```python
from build123d import *

# Parameters (mm, degrees)
SKETCH_3_W           = 2
SKETCH_3_H           = 46.5
SKETCH_5_W           = 2
SKETCH_5_H           = 46.5
SKETCH_6_R           = 9.5
CUT_EXTRUDE_1_DEPTH  = 328.171973127
SKETCH_7_R           = 9.5
CUT_EXTRUDE_2_DEPTH  = 328.171973127
SKETCH_8_R           = 9.5
CUT_EXTRUDE_3_DEPTH  = 328.171973127
SKETCH_9_R           = 9.5
CUT_EXTRUDE_4_DEPTH  = 328.171973127
SKETCH_10_R          = 9.5
CUT_EXTRUDE_5_DEPTH  = 328.171973127
SKETCH_11_R          = 9.5
CUT_EXTRUDE_6_DEPTH  = 328.171973127
SKETCH_12_R          = 9.5
CUT_EXTRUDE_7_DEPTH  = 328.171973127
SKETCH_13_R          = 9.5
CUT_EXTRUDE_8_DEPTH  = 328.171973127
SKETCH_14_R          = 9.5
CUT_EXTRUDE_9_DEPTH  = 328.171973127
SKETCH_15_R          = 9.5
CUT_EXTRUDE_10_DEPTH = 328.171973127
SKETCH_16_R          = 9.5
CUT_EXTRUDE_11_DEPTH = 328.171973127
SKETCH_17_R          = 9.5
CUT_EXTRUDE_12_DEPTH = 328.171973127
SKETCH_18_R          = 6
CUT_EXTRUDE_13_DEPTH = 328.171973127


with BuildPart() as part:
    # Эскиз1 → Повернуть1 (revolve)
    with BuildSketch(Plane.XY, mode=Mode.PRIVATE) as revolve_1_sk:
        with BuildLine():
            Line((0, 0), (273, 0))
            Line((273, 0), (273, 98.4))
            Line((273, 98.4), (271.4, 100))
            Line((271.4, 100), (265, 100))
            Line((265, 100), (265, 127.5))
            Line((265, 127.5), (247, 127.5))
            Line((247, 127.5), (247, 100))
            Line((247, 100), (239, 100))
            Line((239, 100), (239, 62.5))
            Line((239, 62.5), (218, 62.5))
            Line((218, 62.5), (215, 60.767949192))
            Line((215, 60.767949192), (215, 57))
            ThreePointArc((215, 57), (214.414213562, 55.585786438), (213, 55))
            Line((213, 55), (183, 55))
            Line((183, 55), (178.669872981, 52.5))
            Line((178.669872981, 52.5), (95, 52.5))
            Line((95, 52.5), (95, 50))
            Line((95, 50), (42, 50))
            Line((42, 50), (42, 45))
            Line((42, 45), (0, 45))
            Line((0, 45), (0, 0))
        make_face()
    revolve(revolve_1_sk.sketch.rotate(Axis((0, 0, 0), (1, 0, 0)), 90), axis=Axis((0, 0, 0), (1, 0, 0)))

    # Эскиз2 → Вырез-Повернуть1 (revolve, cut)
    with BuildSketch(Plane.XY, mode=Mode.PRIVATE) as cut_revolve_1_sk:
        Polygon((0, 0), (273, 0), (273, 95), (265, 95), (265, 45), (254, 45), (254, 39), (240, 39), (240, 34), (203.5, 34), (203.5, 31), (0, 31), align=None)
    revolve(cut_revolve_1_sk.sketch.rotate(Axis((0, 0, 0), (1, 0, 0)), 90), axis=Axis((0, 0, 0), (1, 0, 0)), mode=Mode.SUBTRACT)

    # Эскиз3 → Rear_recess_left (revolve, cut)
    with BuildSketch(Plane.XY, mode=Mode.PRIVATE) as rear_recess_left_sk:
        with Locations((261, 71.75)):
            Rectangle(SKETCH_3_W, SKETCH_3_H)
    revolve(rear_recess_left_sk.sketch.rotate(Axis((0, 0, 0), (1, 0, 0)), 90), axis=Axis((0, 0, 0), (1, 0, 0)), mode=Mode.SUBTRACT)

    # Эскиз4 → Collar_groove_nominal (revolve, cut)
    with BuildSketch(Plane.XY, mode=Mode.PRIVATE) as collar_groove_nominal_sk:
        with BuildLine():
            Line((263, 48), (263, 95))
            Line((263, 95), (262, 95))
            Line((262, 95), (262, 48))
            ThreePointArc((262, 48), (262.146446609, 47.646446609), (262.5, 47.5))
            ThreePointArc((262.5, 47.5), (262.853553391, 47.646446609), (263, 48))
        make_face()
    revolve(collar_groove_nominal_sk.sketch.rotate(Axis((0, 0, 0), (1, 0, 0)), 90), axis=Axis((0, 0, 0), (1, 0, 0)), mode=Mode.SUBTRACT)

    # Эскиз5 → Rear_recess_lip (revolve, cut)
    with BuildSketch(Plane.XY, mode=Mode.PRIVATE) as rear_recess_lip_sk:
        with Locations((264, 71.75)):
            Rectangle(SKETCH_5_W, SKETCH_5_H)
    revolve(rear_recess_lip_sk.sketch.rotate(Axis((0, 0, 0), (1, 0, 0)), 90), axis=Axis((0, 0, 0), (1, 0, 0)), mode=Mode.SUBTRACT)

    # Эскиз6 → Вырез-Вытянуть1 (cut, through all)
    with BuildSketch(Plane(origin=(0, 0, 0), x_dir=(0, 0, -1), z_dir=(1, 0, 0))):
        with Locations(Location((0, 113, 0), (0, 0, 180))):
            Circle(SKETCH_6_R)
    extrude(amount=CUT_EXTRUDE_1_DEPTH, mode=Mode.SUBTRACT)

    # Эскиз7 → Вырез-Вытянуть2 (cut, through all)
    with BuildSketch(Plane(origin=(0, 0, 0), x_dir=(0, 0, -1), z_dir=(1, 0, 0))):
        with Locations(Location((-56.5, 97.860870628, 0), (0, 0, 180))):
            Circle(SKETCH_7_R)
    extrude(amount=CUT_EXTRUDE_2_DEPTH, mode=Mode.SUBTRACT)

    # Эскиз8 → Вырез-Вытянуть3 (cut, through all)
    with BuildSketch(Plane(origin=(0, 0, 0), x_dir=(0, 0, -1), z_dir=(1, 0, 0))):
        with Locations(Location((-97.860870628, 56.5, 0), (0, 0, 180))):
            Circle(SKETCH_8_R)
    extrude(amount=CUT_EXTRUDE_3_DEPTH, mode=Mode.SUBTRACT)

    # Эскиз9 → Вырез-Вытянуть4 (cut, through all)
    with BuildSketch(Plane(origin=(0, 0, 0), x_dir=(0, 0, -1), z_dir=(1, 0, 0))):
        with Locations(Location((-113, 0, 0), (0, 0, 180))):
            Circle(SKETCH_9_R)
    extrude(amount=CUT_EXTRUDE_4_DEPTH, mode=Mode.SUBTRACT)

    # Эскиз10 → Вырез-Вытянуть5 (cut, through all)
    with BuildSketch(Plane(origin=(0, 0, 0), x_dir=(0, 0, -1), z_dir=(1, 0, 0))):
        with Locations(Location((-97.860870628, -56.5, 0), (0, 0, 180))):
            Circle(SKETCH_10_R)
    extrude(amount=CUT_EXTRUDE_5_DEPTH, mode=Mode.SUBTRACT)

    # Эскиз11 → Вырез-Вытянуть6 (cut, through all)
    with BuildSketch(Plane(origin=(0, 0, 0), x_dir=(0, 0, -1), z_dir=(1, 0, 0))):
        with Locations(Location((-56.5, -97.860870628, 0), (0, 0, 180))):
            Circle(SKETCH_11_R)
    extrude(amount=CUT_EXTRUDE_6_DEPTH, mode=Mode.SUBTRACT)

    # Эскиз12 → Вырез-Вытянуть7 (cut, through all)
    with BuildSketch(Plane(origin=(0, 0, 0), x_dir=(0, 0, -1), z_dir=(1, 0, 0))):
        with Locations(Location((0, -113, 0), (0, 0, 180))):
            Circle(SKETCH_12_R)
    extrude(amount=CUT_EXTRUDE_7_DEPTH, mode=Mode.SUBTRACT)

    # Эскиз13 → Вырез-Вытянуть8 (cut, through all)
    with BuildSketch(Plane(origin=(0, 0, 0), x_dir=(0, 0, -1), z_dir=(1, 0, 0))):
        with Locations(Location((56.5, -97.860870628, 0), (0, 0, 180))):
            Circle(SKETCH_13_R)
    extrude(amount=CUT_EXTRUDE_8_DEPTH, mode=Mode.SUBTRACT)

    # Эскиз14 → Вырез-Вытянуть9 (cut, through all)
    with BuildSketch(Plane(origin=(0, 0, 0), x_dir=(0, 0, -1), z_dir=(1, 0, 0))):
        with Locations(Location((97.860870628, -56.5, 0), (0, 0, 180))):
            Circle(SKETCH_14_R)
    extrude(amount=CUT_EXTRUDE_9_DEPTH, mode=Mode.SUBTRACT)

    # Эскиз15 → Вырез-Вытянуть10 (cut, through all)
    with BuildSketch(Plane(origin=(0, 0, 0), x_dir=(0, 0, -1), z_dir=(1, 0, 0))):
        with Locations(Location((113, 0, 0), (0, 0, 180))):
            Circle(SKETCH_15_R)
    extrude(amount=CUT_EXTRUDE_10_DEPTH, mode=Mode.SUBTRACT)

    # Эскиз16 → Вырез-Вытянуть11 (cut, through all)
    with BuildSketch(Plane(origin=(0, 0, 0), x_dir=(0, 0, -1), z_dir=(1, 0, 0))):
        with Locations(Location((97.860870628, 56.5, 0), (0, 0, 180))):
            Circle(SKETCH_16_R)
    extrude(amount=CUT_EXTRUDE_11_DEPTH, mode=Mode.SUBTRACT)

    # Эскиз17 → Вырез-Вытянуть12 (cut, through all)
    with BuildSketch(Plane(origin=(0, 0, 0), x_dir=(0, 0, -1), z_dir=(1, 0, 0))):
        with Locations(Location((56.5, 97.860870628, 0), (0, 0, 180))):
            Circle(SKETCH_17_R)
    extrude(amount=CUT_EXTRUDE_12_DEPTH, mode=Mode.SUBTRACT)

    # Эскиз18 → Вырез-Вытянуть13 (cut, through all)
    with BuildSketch(Plane(origin=(0, 0, 0), x_dir=(0, 0, -1), z_dir=(1, 0, 0))):
        with Locations((0, -84)):
            Circle(SKETCH_18_R)
    extrude(amount=CUT_EXTRUDE_13_DEPTH, mode=Mode.SUBTRACT)


solid = part.part
```
Here's how the part is built. I have some questions about the finished solid (model axes, mm). A direction names the side the tool comes from. Give positions to 0.01 mm unless a question says otherwise; leave off trailing zeros. Loops run counter-clockwise (first coordinate to the right, second up) from the corner with the lowest first, then second, coordinate; pieces in that order, holes last. Notation, with made-up numbers: (54.25, -7) -> (76.25, -7) arc R19 cw to (76.25, 5) -> close; hole circle Ø11 at (47, 78). An arc over 180 degrees is marked (long way). Use one line per item in the form item = value. Start each with the question number.
1) Imagine slicing it at D-D (x = 148). Please give me the cut outline in (y, z).
2) Imagine slicing it at A-A (z = 113). Please give me the cut outline in (x, y), then the cut area to 3 significant figures.
3) For P1, Ø1.5, axis at x = 35, z = 3.5, coming from the +Y side; P2, Ø24.5, axis at y = 56.5, z = -97.86, coming from the +X side; P3, Ø1, axis at x = 220, z = 6.5, coming from the -Y side; P4, Ø11.5, axis at y = -97.86, z = -56.5, coming from the -X side, each with a flat end and sliding along its axis, tell me the tip position at first contact or that it passes through.
4) Imagine slicing it at B-B (x = 85.5). Please give me the cut outline in (y, z), then the cut area to 3 significant figures.
5) Please list where these lines run through material, in increasing order: line 1 along Y through (x, z) = (258.5, 0); line 2 along Y through (x, z) = (254.5, 56.5); line 3 along Z through (x, y) = (253.5, -65).
6) Thinking about a two-plate mould opening in Y: for faces 1 (the face through (265, 43, 14)), 2 (the face through (215, -54.3, -18.3)), 3 (the face through (242.94, -30.04, 95.38)), which applies, +Y half, -Y half, draft (parallel to the pull), parting line (faces both ways), or undercut?
7) Which directions (+Z, -Z, +X, -X, +Y, -Y) give clear straight access to the entire face, cutting with the end or side of a thin tool? Please do faces 4 (the face through (197.79, 48.794, 25.379)), 5 (the face through (221.49, -33.71, -4.43)), 6 (the face through (249.35, -78.05, 0.78)).
Check values:
q1.outline = circle Ø105 at (0, 0); hole circle Ø62 at (0, 0)
q2.outline = (247, -59.05) -> (265, -59.05) -> (265, -9.5) -> (247, -9.5) -> close; (247, 9.5) -> (265, 9.5) -> (265, 59.05) -> (247, 59.05) -> close
q2.area = 1,780 mm^2
q3.P1 = 44.92
q3.P2 = 265
q3.P3 = -62.21
q3.P4 = through
q4.outline = circle Ø100 at (0, 0); hole circle Ø62 at (0, 0)
q4.area = 4,830 mm^2
q5.line_1 = -127.5 to -122.5, -103.5 to -90, -78 to -45, 45 to 103.5, 122.5 to 127.5
q5.line_2 = -114.3 to -107.36, -88.36 to 88.36, 107.36 to 114.3
q5.line_3 = -109.69 to -102.1, -93.62 to 93.62, 102.1 to 109.69
q6.face_1 = undercut
q6.face_2 = draft
q6.face_3 = parting line
q7.face_4 = -X
q7.face_5 = +X
q7.face_6 = +X, -X
